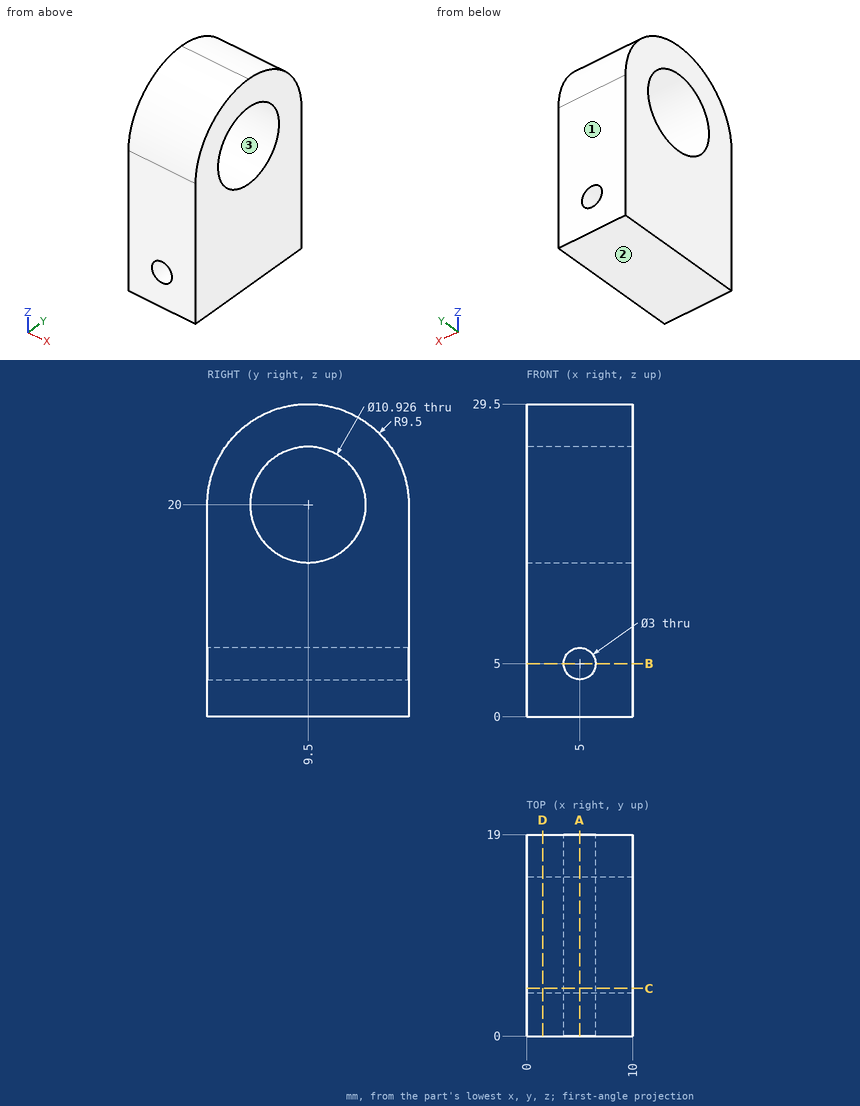
For this review, use the dimensioned drawing (mm, ordinates from the lowest corner) and the shaded views. Round coordinates to 2 decimals unless told otherwise and drop trailing zeros. Order: outer loops, then holes, each group sorted by start corner. A loop starts at its lowest first (then second) coordinate and runs counter-clockwise, first axis right, second up. Notation, with made-up numbers: (-22, -31.75) -> (7, -31.75) arc R14 cw to (7, -4.75) -> close; hole circle Ø5 at (-29.75, 79). An arc over 180 degrees is marked (long way). Write item = value, one per line. Start each with the question number.
Item 1: Consider section B-B on z = 5. Write out the cut boundary in (x, y).
Item 2: Mouldability with a two-part tool opening along Y and no side actions: class the marked faces 1, 2 and 3 as released by +Y, released by -Y, zero draft, split by the parting line, or undercut.
Item 3: Consider section D-D on x = 1.5. Write out the cut boundary in (y, z).
Item 4: For line 1 along X through (y, z) = (4.75, 5); line 2 along Z through (x, y) = (6, 11); line 3 along Y through (x, z) = (5, 20), list the stretches that pass through material, from the lowest coordinate up.
Item 5: Consider section C-C on y = 4.5. Write out the cut boundary in (x, z), plus the area to 3 significant figures.
Item 6: Consider section A-A on x = 5. Write out the cut boundary in (y, z), plus the area to 3 significant figures.
Item 7: Clearance check with a flat-ended pin moving along its axis: pin 1 Ø3 at (y, z) = (8.5, 16.5) entering from +X. State where the tip first meets the part, or that it passes through.
Conclusion:
q1.outline = (0, 0) -> (3.5, 0) -> (3.5, 19) -> (0, 19) -> close; (6.5, 0) -> (10, 0) -> (10, 19) -> (6.5, 19) -> close
q2.face_1 = released by +Y
q2.face_2 = zero draft
q2.face_3 = undercut
q3.outline = (0, 0) -> (19, 0) -> (19, 20) arc R9.5 ccw to (0, 20) -> close; hole circle Ø10.93 at (9.5, 20)
q4.line_1 = 0 to 3.5, 6.5 to 10
q4.line_2 = 0 to 3.88, 6.12 to 14.75, 25.25 to 29.38
q4.line_3 = 0 to 4.04, 14.96 to 19
q5.outline = (0, 0) -> (10, 0) -> (10, 17.8) -> (0, 17.8) -> close; (0, 22.2) -> (10, 22.2) -> (10, 28.08) -> (0, 28.08) -> close; hole circle Ø3 at (5, 5)
q5.area = 230 mm2
q6.outline = (0, 0) -> (19, 0) -> (19, 3.5) -> (0, 3.5) -> close; (0, 6.5) -> (19, 6.5) -> (19, 20) arc R9.5 ccw to (0, 20) -> close; hole circle Ø10.93 at (9.5, 20)
q6.area = 371 mm2
q7.pin_1 = through
